```python
from build123d import *

# Parameters (mm, degrees)
SKETCH1_W             = 19.05
SKETCH1_H             = 19.05
BOSS_EXTRUDE1_DEPTH   = 254
SKETCH3_W             = 2.4892
SKETCH3_H             = 19.05
SKETCH3_AT_POINT_2_W  = 2.4892
SKETCH3_AT_POINT_2_H  = 19.05
LPATTERN1_START       = -11
LPATTERN1_OUTLINE_R   = 2.4892
LPATTERN1_DEPTH       = 22
LPATTERN1_2_OUTLINE_R = 2.4892
LPATTERN1_2_DEPTH     = 22


with BuildPart() as part:
    # Sketch1 → Boss-Extrude1 (new, symmetric)
    with BuildSketch(Plane(origin=(0, 0, 0), x_dir=(0, 0, -1), z_dir=(1, 0, 0))):
        Rectangle(SKETCH1_W, SKETCH1_H)
    extrude(amount=BOSS_EXTRUDE1_DEPTH, both=True)

    # Sketch3 → #9 (0.196) Diameter Hole1 (revolve, cut)
    with BuildSketch(Plane(origin=(241.3, 9.525, 0), x_dir=(0, 0, 1), z_dir=(1, 0, 0))):
        with Locations((1.2446, 9.525)):
            Rectangle(SKETCH3_W, SKETCH3_H)
    revolve(axis=Axis((241.3, 15.875, 0), (0, -1, 0)), mode=Mode.SUBTRACT)

    # Sketch3 at point 2 (carried to point 2, square into its face) → #9 (0.196) Diameter Hole1 at 2 (revolve, cut)
    with BuildSketch(Plane(origin=(241.3, 0, 9.525), x_dir=(0, -1, 0), z_dir=(1, 0, 0))):
        with Locations((1.2446, 9.525)):
            Rectangle(SKETCH3_AT_POINT_2_W, SKETCH3_AT_POINT_2_H)
    revolve(axis=Axis((241.3, 0, 15.875), (0, 0, -1)), mode=Mode.SUBTRACT)

    # LPattern1: read off the stored shape, not the designer's step
    # LPattern1 outline → LPattern1 (cut)
    with BuildSketch(Plane.XY.offset(LPATTERN1_START)):
        with Locations((-241.3, 0)):
            Circle(LPATTERN1_OUTLINE_R)
        with Locations((-215.9, 0)):
            Circle(LPATTERN1_OUTLINE_R)
        with Locations((-190.5, 0)):
            Circle(LPATTERN1_OUTLINE_R)
        with Locations((-165.1, 0)):
            Circle(LPATTERN1_OUTLINE_R)
        with Locations((-139.7, 0)):
            Circle(LPATTERN1_OUTLINE_R)
        with Locations((-114.3, 0)):
            Circle(LPATTERN1_OUTLINE_R)
        with Locations((-88.9, 0)):
            Circle(LPATTERN1_OUTLINE_R)
        with Locations((-63.5, 0)):
            Circle(LPATTERN1_OUTLINE_R)
        with Locations((-38.1, 0)):
            Circle(LPATTERN1_OUTLINE_R)
        with Locations((-12.7, 0)):
            Circle(LPATTERN1_OUTLINE_R)
        with Locations((12.7, 0)):
            Circle(LPATTERN1_OUTLINE_R)
        with Locations((38.1, 0)):
            Circle(LPATTERN1_OUTLINE_R)
        with Locations((63.5, 0)):
            Circle(LPATTERN1_OUTLINE_R)
        with Locations((88.9, 0)):
            Circle(LPATTERN1_OUTLINE_R)
        with Locations((114.3, 0)):
            Circle(LPATTERN1_OUTLINE_R)
        with Locations((139.7, 0)):
            Circle(LPATTERN1_OUTLINE_R)
        with Locations((165.1, 0)):
            Circle(LPATTERN1_OUTLINE_R)
        with Locations((190.5, 0)):
            Circle(LPATTERN1_OUTLINE_R)
        with Locations((215.9, 0)):
            Circle(LPATTERN1_OUTLINE_R)
    extrude(amount=LPATTERN1_DEPTH, mode=Mode.SUBTRACT)

    # LPattern1 2 outline → LPattern1 2 (cut)
    with BuildSketch(Plane(origin=(0, 0, 0), x_dir=(1, 0, 0), z_dir=(0, 1, 0)).offset(LPATTERN1_START)):
        with Locations((215.9, 0)):
            Circle(LPATTERN1_2_OUTLINE_R)
        with Locations((190.5, 0)):
            Circle(LPATTERN1_2_OUTLINE_R)
        with Locations((165.1, 0)):
            Circle(LPATTERN1_2_OUTLINE_R)
        with Locations((139.7, 0)):
            Circle(LPATTERN1_2_OUTLINE_R)
        with Locations((114.3, 0)):
            Circle(LPATTERN1_2_OUTLINE_R)
        with Locations((88.9, 0)):
            Circle(LPATTERN1_2_OUTLINE_R)
        with Locations((63.5, 0)):
            Circle(LPATTERN1_2_OUTLINE_R)
        with Locations((38.1, 0)):
            Circle(LPATTERN1_2_OUTLINE_R)
        with Locations((12.7, 0)):
            Circle(LPATTERN1_2_OUTLINE_R)
        with Locations((-12.7, 0)):
            Circle(LPATTERN1_2_OUTLINE_R)
        with Locations((-38.1, 0)):
            Circle(LPATTERN1_2_OUTLINE_R)
        with Locations((-63.5, 0)):
            Circle(LPATTERN1_2_OUTLINE_R)
        with Locations((-88.9, 0)):
            Circle(LPATTERN1_2_OUTLINE_R)
        with Locations((-114.3, 0)):
            Circle(LPATTERN1_2_OUTLINE_R)
        with Locations((-139.7, 0)):
            Circle(LPATTERN1_2_OUTLINE_R)
        with Locations((-165.1, 0)):
            Circle(LPATTERN1_2_OUTLINE_R)
        with Locations((-190.5, 0)):
            Circle(LPATTERN1_2_OUTLINE_R)
        with Locations((-215.9, 0)):
            Circle(LPATTERN1_2_OUTLINE_R)
        with Locations((-241.3, 0)):
            Circle(LPATTERN1_2_OUTLINE_R)
    extrude(amount=LPATTERN1_2_DEPTH, mode=Mode.SUBTRACT)


solid = part.part
```
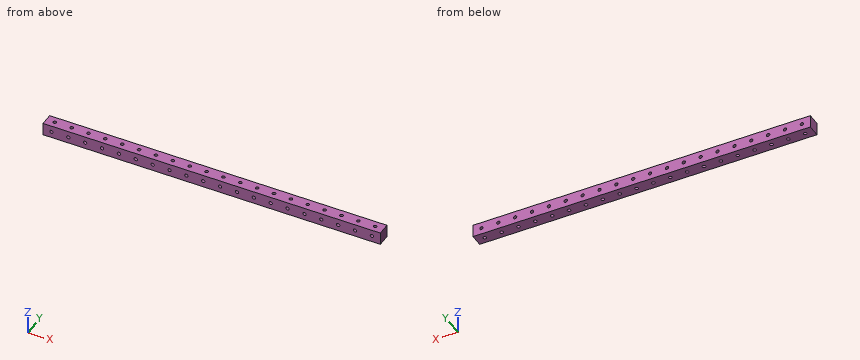
Input: part model. Units: mm. Frame: model coordinates. Round coordinates to 2 decimals unless told otherwise and drop trailing zeros. Answer as CSV lines item,"result".
1. Section A-A (z = 5.5). Give the number of separate pieces and of enclosed holes in the cut face, plus the area to 3 significant figures.
Geometry says:
separate pieces,"1"
enclosed holes,"20"
area,"9,290 mm^2"
2. Contact query for flat-ended pins moving along their axis: P1, Ø6.5, axis at x = -12.7, y = 0, coming from the +Z side (3 decimals); P2, Ø4.5, axis at x = 190.5, z = 0, coming from the -Y side. Output: stop coordinate, or through.
Geometry says:
P1,"stops at z = 9.525"
P2,"passes through"
3. Ray query, L1, parallel to Y at x = 64, z = 5 (3 decimals); L2, parallel to Y at x = -139.7, z = -3 (3 decimals). Return the intervals inside material, ascending. Write a range as [from, to].
Geometry says:
L1,"y = [-9.525, -2.438], [2.438, 9.525]"
L2,"y = [-9.525, -2.489], [2.489, 9.525]"
